Can you work these out from the model? Positions are in its coordinate system, mm. A direction names the side the tool comes from. Coordinates: 2 decimals unless noted, no trailing zeros. Order: outer loops, then holes, each group sorted by start corner. A loop starts at its lowest first (then second) coordinate and runs counter-clockwise, first axis right, second up. Notation, with made-up numbers: (-5, 51) -> (43, 51) arc R29 ccw to (43, 75) -> close; hole circle Ø7 at (51, -34). An arc over 180 degrees is marked (long way). Answer in a Markdown table with one row per item. Add a question column.
1. Imagine slicing it at D-D on z = 4.3. Write out the boundary of the cut face in (x, y).
2. Imagine slicing it at C-C on z = 1. Write out the boundary of the cut face in (x, y), plus the area to 3 significant figures.
3. If I drill on line 1 along Z through (x, y) = (-3.5, 3); line 2 along Z through (x, y) = (0.75, -1.75); line 3 along X through (y, z) = (0.5, 1.1), over which ranges is the centre line in solid material (lowest first)? Write a range as [from, to].
4. Will these pins go through, and if not, where does the flat tip stop? pin 1 (1.5 mm diameter, centred on y = 1.5, z = 4.5, fed in from -X); pin 2 (2.5 mm diameter, centred on x = -1, y = 0, fed in from -Z).
5. On a 3-axis mill with a long thin cutter (end or side, diameter ignored), from which of +Z, -Z, +X, -X, +Y, -Y can I reach the whole of each face in a straight line? I mean faces 1 (the face through (-2, -2, 0)), 2 (the face through (-2, -2, 3.2)), 3 (the face through (0, 0, 1.7)). Say none if no direction works.
6. Imagine slicing it at A-A on x = 0. Write out the boundary of the cut face in (y, z).
Autodesk Inventor part; units mm, degrees
ref_plane "YZ Plane" through (0, 0, 0) normal (1, 0, 0) x (0, 1, 0)
ref_plane "XZ Plane" through (0, 0, 0) normal (0, 1, 0) x (-1, 0, 0)
ref_plane "XY Plane" through (0, 0, 0) normal (0, 0, 1) x (1, 0, 0)
sketch "Sketch1" plane through (0, 0, 0) normal (0, 0, 1) x (1, 0, 0)
  line L0 (-4, -4) -> (4, -4)
  line L1 (4, -4) -> (4, 4)
  line L2 (4, 4) -> (-4, 4)
  line L3 (-4, 4) -> (-4, -4)
  line L4 (-4, -4) -> (4, 4) construction
  line L5 (4, -4) -> (-4, 4) construction
  circle A0 centre (0, 0) radius 2.4
  dimension "d0" = 8
  dimension "d1" = 8
  dimension "d2" = 4.8
extrude "Extrusion1" add sketch "Sketch1" along normal blind 3.2 contours L3 L2 L1 L0 | A0
extrude "Extrusion2" add sketch "Sketch1" along normal blind 4.9 contours A0
extrude "Extrusion3" cut sketch "Sketch1" along normal blind 1.7 contours A0
pattern_of_one "Rectangular Pattern1"
equation "\"d11\" = d0"
equation "\"d24\" = d0"
properties part number "LEGO Stud 1x1 Transparent Dark Blue"
Answers follow:
| question | item | result |
|---|---|---|
| 1 | outline | circle Ø4.8 at (0, 0) |
| 2 | outline | (-4, -4) -> (4, -4) -> (4, 4) -> (-4, 4) -> close; hole circle Ø4.8 at (0, 0) |
| 2 | area | 45.9 mm² |
| 3 | line 1 | z = [0, 3.2] |
| 3 | line 2 | z = [1.7, 4.9] |
| 3 | line 3 | x = [-4, -2.35], [2.35, 4] |
| 4 | pin 1 | stops at x = -2.28 |
| 4 | pin 2 | stops at z = 1.7 |
| 5 | face 1 | -Z, +X, -X, +Y, -Y |
| 5 | face 2 | +Z |
| 5 | face 3 | -Z |
| 6 | outline | (-4, 0) -> (-2.4, 0) -> (-2.4, 1.7) -> (2.4, 1.7) -> (2.4, 0) -> (4, 0) -> (4, 3.2) -> (2.4, 3.2) -> (2.4, 4.9) -> (-2.4, 4.9) -> (-2.4, 3.2) -> (-4, 3.2) -> close |
